from build123d import *

# Parameters (mm, degrees)
F0_W     = 34.925
F0_H     = 8.9647058824
F1_DEPTH = 8.9647058824
F2_W     = 6.9327058824
F2_H     = 7.9487058824
F3_DEPTH = 34.926
F4_W     = 2.0463057544
F4_H     = 6.9543164351
F5_DEPTH = 11.1125


# Not quite as in the source:
# - a length typed as a fraction of an inch, garbled in the dataset ("3 / 203.2 mm" for 3/8 in), is restored


with BuildPart() as f1:
    # F0 (on Top) → F1 (new body)
    with BuildSketch(Plane.XY):
        with Locations((-7.0361781826, 4.5039634939)):
            Rectangle(F0_W, F0_H)
    extrude(amount=F1_DEPTH)

    # F2 (on face) → F3 (cut, through all)
    with BuildSketch(Plane.YZ.offset(10.4263218174)):
        with Locations((4.5039634939, 3.9743529412)):
            Rectangle(F2_W, F2_H)
    extrude(amount=-F3_DEPTH, mode=Mode.SUBTRACT)

    # F4 (on face) → F5 (join)
    with BuildSketch(Plane.XY.offset(8.9647058824)):
        with BuildLine():
            ThreePointArc((5.6638218174, 1.016), (7.1045145349, 4.4931582176), (5.6638218174, 7.9703164351))
            Line((5.6638218174, 7.9703164351), (5.6638218174, 1.016))
        make_face()
        with Locations((4.6406689402, 4.4931582176)):
            Rectangle(F4_W, F4_H)
    extrude(amount=F5_DEPTH)


solid = f1.part
Model file for the job. Use its own axes, mm. A direction names the side the tool comes from. Give positions to 0.01 mm unless a question says otherwise; leave off trailing zeros. Write each loop counter-clockwise with the first axis right and the second up, starting at its lowest first coordinate (ties: lowest second). Pieces come first, ordered by that corner, then holes. Notation, with made-up numbers: M 55.5,-32 L 104.5,-32 A26 ccw 104.5,5 Z; hole C -15,73 d2. An arc over 180 degrees is marked long. One line per item, written item: value. Start each with the question number.
Q1. Saw through at C-C, the plane y = 5.5. Write the cut outline in (x, z), plus the area to 3 significant figures.
Q2. Drop flat-ended pins along their axis: pin 1 Ø1.5 at (y, z) = (8, 14.5) entering from +X; pin 2 Ø1 at (x, z) = (4.5, 17) entering from +Y; pin 3 Ø2 at (y, z) = (1.5, 11) entering from +X. Give the stop position or say it passes through.
Q3. 3-axis set-ups, long thin cutter, end or side, ignore diameter. For faces 4 (the flat face through (-7, 1.038, 4)), 5 (the cylindrical face through (7.104, 4.439, 14.443)), 6 (the flat face through (3.618, 4, 14)), 7 (the flat face through (5, 1.016, 14)): which of +Z, -Z, +X, -X, +Y, -Y reach the whole face in a straight line?
Q4. Probe probe 1 along Y at (x, z) = (-4.5, 2.75); probe 2 along Y at (x, z) = (4, 15.5); probe 3 along Z at (x, y) = (-14, 4). List the from-to ranges inside material, lowest first. Write a range as [from, to].
Q5. Two-plate mould, pull along Y, no slides. Class faces 1 (the flat face through (-7, 4, 7.949)), 2 (the flat face through (5, 7.97, 14)), 3 (the flat face through (-7.3, 0.5, 0)): +Y half, -Y half, draft (parallel to the pull), parting line (faces both ways), or undercut.
Q6. Saw through at D-D, the plane z = 16.75. Write the cut outline in (x, y), plus the area to 3 significant figures.
Q7. Saw through at A-A, the plane z = 2. Write the cut outline in (x, y).
Q8. Saw through at B-B, the plane x = -9. Write the cut outline in (y, z).
Output values:
1. outline: M -24.5,7.95 L 10.43,7.95 L 10.43,8.96 L 7,8.96 L 7,20.08 L 3.62,20.08 L 3.62,8.96 L -24.5,8.96 Z
1. area: 73.1 mm²
2. pin 1: stops at x = 6.26
2. pin 2: stops at y = 7.97
2. pin 3: stops at x = 6.68
3. face 4: -Z, +X, -X
3. face 5: +Z, +X
3. face 6: +Z, -X, +Y, -Y
3. face 7: +Z, +X, -X, -Y
4. probe 1: y = [0.02, 1.04], [7.97, 8.99]
4. probe 2: y = [1.02, 7.97]
4. probe 3: z = [7.95, 8.96]
5. face 1: undercut
5. face 2: +Y half
5. face 3: draft
6. outline: M 3.62,1.02 L 5.66,1.02 A4.92 ccw 5.66,7.97 L 3.62,7.97 Z
6. area: 21.1 mm²
7. outline: M -24.5,0.02 L 10.43,0.02 L 10.43,1.04 L -24.5,1.04 Z; M -24.5,7.97 L 10.43,7.97 L 10.43,8.99 L -24.5,8.99 Z
8. outline: M 0.02,0 L 1.04,0 L 1.04,7.95 L 7.97,7.95 L 7.97,0 L 8.99,0 L 8.99,8.96 L 0.02,8.96 Z
